Geometry: final body of the model. Coordinates: model frame, mm. Give positions to 0.01 mm unless a question says otherwise; leave off trailing zeros. Write each loop counter-clockwise with the first axis right and the second up, starting at its lowest first coordinate (ties: lowest second). Pieces come first, ordered by that corner, then holes. Notation, with made-up numbers: (4.25, -20) -> (45.25, -20) arc R24 cw to (45.25, 12) -> close; hole circle Ø8 at (-13.5, 33.5). An arc over 180 degrees is marked (long way). Answer in a Markdown table with one row per item. Add a question column.
from build123d import *

# Parameters (mm, degrees)
F0_W     = 44.358856976
F0_H     = 12.7014997415
F1_DEPTH = 1.5
F2_R     = 1.5


# Not quite as in the source:
# - a feature names something its author has since deleted; it is built from what else it names


with BuildPart() as f1:
    # F0 (on Top) → F1 (new body, symmetric)
    with BuildSketch(Plane.XY):
        with Locations((10.1427063346, 0.782278832)):
            Rectangle(F0_W, F0_H)
        with BuildLine():
            ThreePointArc((-12.0367221534, 7.1330287028), (-18.3874720242, 0.782278832), (-12.0367221534, -5.5684710387))
            Line((-12.0367221534, -5.5684710387), (-12.0367221534, 7.1330287028))
        make_face()
        with BuildLine():
            Line((32.3221348226, 7.1330287028), (32.3221348226, -5.5684710387))
            ThreePointArc((32.3221348226, -5.5684710387), (38.6728846934, 0.782278832), (32.3221348226, 7.1330287028))
        make_face()
    extrude(amount=F1_DEPTH, both=True)

    # F2
    f2_edges = [f1.edges().sort_by_distance(p)[0] for p in [
        (10.142706, -5.568471, 1.5),
        (10.142706, 7.133029, 1.5),
        (38.672885, 0.782279, 1.5),
    ]]
    fillet(f2_edges, radius=F2_R)


solid = f1.part
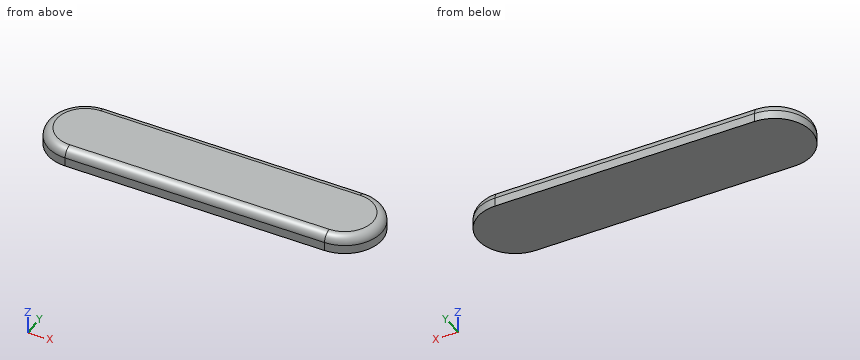
Q1. Line query: probe 1 along X at (y, z) = (2.75, 0.4); probe 2 along X at (y, z) = (-4.25, 0.8); probe 3 along Y at (x, z) = (17.5, 1.2). Output: solid intervals per line, ascending. Write a range as from..to.
Q2. Section A-A on x = 26.5. Return loops of the section in (y, z).
Q3. Contact query for a flat-ended pin moving along its axis: pin 1 Ø1 at (y, z) = (0, 1) entering from -X. Output: stop coordinate, or through.
Q4. Section B-B on z = -0.7. Return loops of the section in (x, y), and give its area (3 significant figures).
Checks:
| question | item | result |
|---|---|---|
| 1 | probe 1 | -18.02..38.3 |
| 1 | probe 2 | -15.52..35.8 |
| 1 | probe 3 | -4.97..6.53 |
| 2 | outline | (-5.57, -1.5) -> (7.13, -1.5) -> (7.13, 0) arc R1.5 ccw to (5.63, 1.5) -> (-4.07, 1.5) arc R1.5 ccw to (-5.57, 0) -> close |
| 3 | pin 1 | x = -18.26 |
| 4 | outline | (-12.04, -5.57) -> (32.32, -5.57) arc R6.35 ccw to (32.32, 7.13) -> (-12.04, 7.13) arc R6.35 ccw to start |
| 4 | area | 690 mm^2 |
